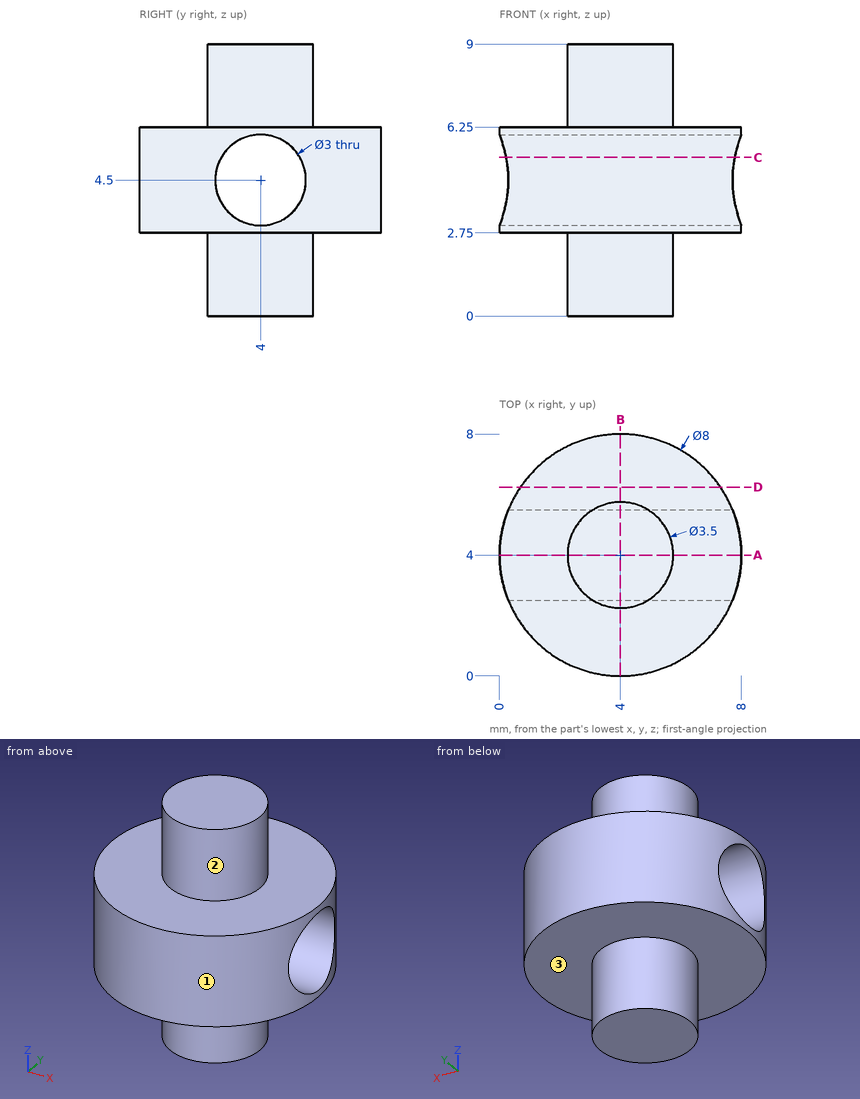
The drawing under review shows one solid part. Ordinate dimensions are in mm from its lowest x, y, z. A direction names the side the tool comes from. Give positions to 0.01 mm unless a question says otherwise; leave off trailing zeros. Order: outer loops, then holes, each group sorted by start corner. A loop starts at its lowest first (then second) coordinate and runs counter-clockwise, first axis right, second up. Notation, with made-up numbers: (42, -24) -> (48, -24) arc R14 ccw to (48, -17) -> close; hole circle Ø8 at (-34, 17.5). An arc over 180 degrees is marked (long way). Write item = value, one per line.
1) We need section A-A, the plane y = 4. Give the boundary of the cut face in (x, z).
Findings:
outline = (0, 2.75) -> (2.25, 2.75) -> (2.25, 0) -> (5.75, 0) -> (5.75, 2.75) -> (8, 2.75) -> (8, 3) -> (0, 3) -> close; (0, 6) -> (8, 6) -> (8, 6.25) -> (5.75, 6.25) -> (5.75, 9) -> (2.25, 9) -> (2.25, 6.25) -> (0, 6.25) -> close
2) Insertion check: pin 1 (2 mm diameter, centred on x = 1.5, z = 3, fed in from -Y); pin 2 (4 mm diameter, centred on x = 1, z = 3, fed in from +Y); pin 3 (3 mm diameter, centred on x = 1, z = 4, fed in from +Y). Each pin has a flat end and moves straight along its axis. Give the tip position at first contact, or say it passes through.
Findings:
pin_1 = 0.29
pin_2 = 7.87
pin_3 = 7.71
3) We need section C-C, the plane z = 5.25. Give the boundary of the cut face in (x, y).
Findings:
outline = (0.22, 2.7) arc R4 ccw to (7.78, 2.7) -> close; (0.22, 5.3) -> (7.78, 5.3) arc R4 ccw to start
4) To check wall thickness, follow L1, parallel to Z at x = 2.75, y = 4; L2, parallel to Z at x = 2.5, y = 2.75; L3, parallel to Y at x = 6.75, z = 4.5. State the ranges of each line that lie inside material, in increasing order. Write a range as from..to.
Findings:
L1 = 0..3, 6..9
L2 = 2.75..3.67, 5.33..6.25
L3 = 1.1..2.5, 5.5..6.9
5) For the marked faces 1, 2 and 3, list the 3-axis set-ups (+Z, -Z, +X, -X, +Y, -Y) from which the entire face can be reached by the end or side of a thin tool; tool diameter is ignored.
Findings:
face_1 = +Z, -Z
face_2 = +Z
face_3 = -Z
6) We need section D-D, the plane y = 6.25. Give the boundary of the cut face in (x, z), and give its area (3 significant figures).
Findings:
outline = (0.69, 2.75) -> (7.31, 2.75) -> (7.31, 6.25) -> (0.69, 6.25) -> close
area = 23.2 mm^2
7) We need section B-B, the plane x = 4. Give the boundary of the cut face in (y, z).
Findings:
outline = (0, 2.75) -> (2.25, 2.75) -> (2.25, 0) -> (5.75, 0) -> (5.75, 2.75) -> (8, 2.75) -> (8, 6.25) -> (5.75, 6.25) -> (5.75, 9) -> (2.25, 9) -> (2.25, 6.25) -> (0, 6.25) -> close; hole circle Ø3 at (4, 4.5)
